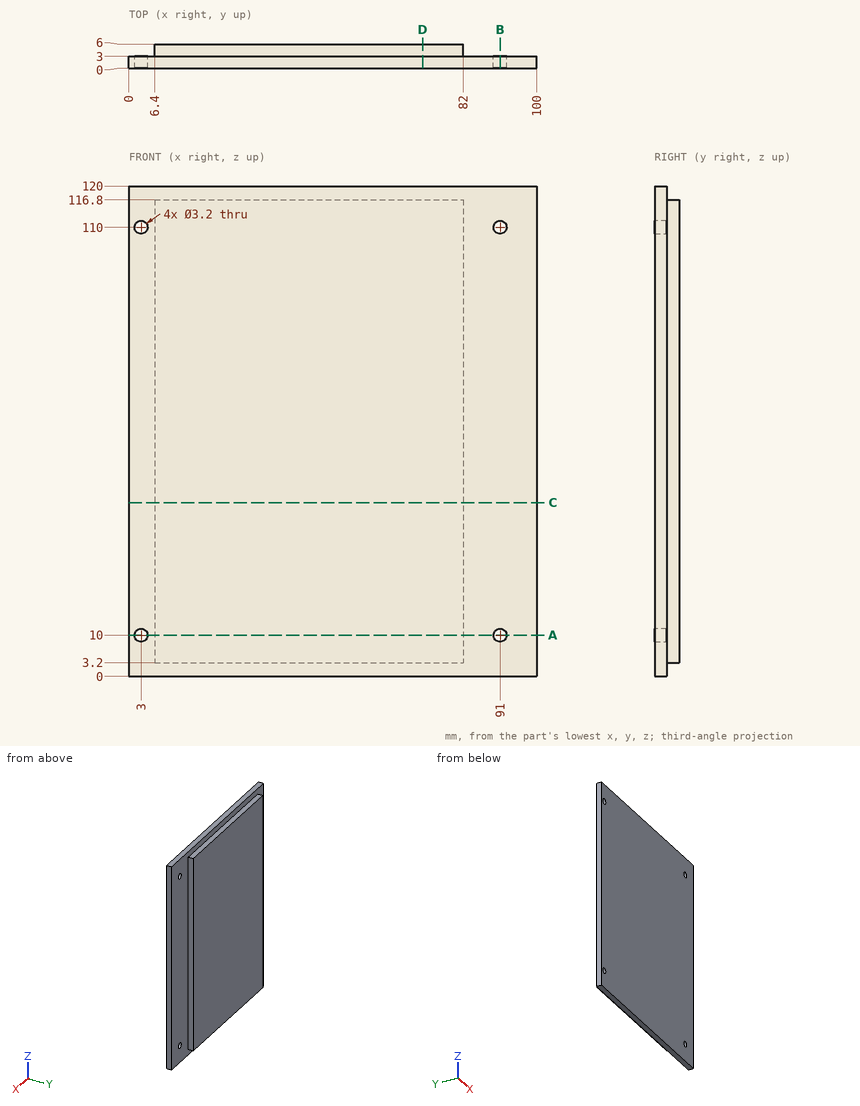
Verification items for this drawing (mm, ordinates from the low corner). Round coordinates to 2 decimals unless told otherwise and drop trailing zeros. Write each loop counter-clockwise with the first axis right and the second up, starting at its lowest first coordinate (ties: lowest second). Pieces come first, ordered by that corner, then holes. Notation, with made-up numbers: (9, 20) - (60, 20) arc R27 cw to (60, 58) - close; hole circle Ø5 at (89, -8). An arc over 180 degrees is marked (long way). One line per item, written item: value.
1. Scan lines: L1, parallel to X at y = 0.8, z = 10; L2, parallel to Z at x = 91, y = 1.3; L3, parallel to X at y = 5, z = 85.5. Record each from-to range of solid material in increasing order.
The answers:
L1: x = 0 to 1.4, 4.6 to 89.4, 92.6 to 100
L2: z = 0 to 8.4, 11.6 to 108.4, 111.6 to 120
L3: x = 6.4 to 82
2. Cross-section at A-A on z = 10. Record the boundary of the cut face in (x, y).
The answers:
outline: (0, 0) - (1.4, 0) - (1.4, 3) - (0, 3) - close; (4.6, 0) - (89.4, 0) - (89.4, 3) - (82, 3) - (82, 6) - (6.4, 6) - (6.4, 3) - (4.6, 3) - close; (92.6, 0) - (100, 0) - (100, 3) - (92.6, 3) - close
3. Cross-section at C-C on z = 42.5. Record the boundary of the cut face in (x, y).
The answers:
outline: (0, 0) - (100, 0) - (100, 3) - (82, 3) - (82, 6) - (6.4, 6) - (6.4, 3) - (0, 3) - close
4. Cross-section at B-B on x = 91. Record the boundary of the cut face in (y, z).
The answers:
outline: (0, 0) - (3, 0) - (3, 8.4) - (0, 8.4) - close; (0, 11.6) - (3, 11.6) - (3, 108.4) - (0, 108.4) - close; (0, 111.6) - (3, 111.6) - (3, 120) - (0, 120) - close
5. Depth check by flat-ended pin: pin 1 Ø0.9 at (x, y) = (53, 5) entering from -Z; pin 2 Ø0.9 at (x, y) = (54.5, 4) entering from +Z. Enter the tip coordinate at first touch or a pass-through.
The answers:
pin 1: stops at z = 3.2
pin 2: stops at z = 116.8
6. Cross-section at D-D on x = 72. Record the boundary of the cut face in (y, z).
The answers:
outline: (0, 0) - (3, 0) - (3, 3.2) - (6, 3.2) - (6, 116.8) - (3, 116.8) - (3, 120) - (0, 120) - close
